from build123d import *

# Parameters (mm, degrees)
MODEL_R         = 1.59999954
EXTRUDE_1_DEPTH = 3.5
SKETCH_2_W      = 135.00000272
SKETCH_2_H      = 6
EXTRUDE_2_DEPTH = 3.5
FILLET_2_R      = 3
FILLET_3_R      = 3
FILLET_4_R      = 3
FILLET_5_R      = 3
FILLET_6_R      = 3
FILLET_7_R      = 3
FILLET_8_R      = 3
FILLET_9_R      = 3
FILLET_10_R     = 3
FILLET_11_R     = 3
FILLET_12_DEPTH = 3.5
FILLET_13_R     = 3
FILLET_14_R     = 3
FILLET_15_DEPTH = 3.5
FILLET_16_R     = 3
FILLET_17_R     = 3
SHELL_5_DEPTH   = 1.55


with BuildPart() as part:
    # Model → 凸台-拉伸1 (new body)
    with BuildSketch(Plane.XY):
        with BuildLine():
            Line((84.889976, 100), (147.00000318, 100))
            ThreePointArc((147.00000318, 100), (149.121322873, 99.121320613), (150.00000226, 97.00000092))
            Line((150.00000226, 97.00000092), (150.00000226, 3.00000162))
            ThreePointArc((150.00000226, 3.00000162), (149.121322873, 0.878681927), (147.00000318, 2.54e-06))
            Line((147.00000318, 2.54e-06), (2.99999908, 2.54e-06))
            ThreePointArc((2.99999908, 2.54e-06), (0.878679387, 0.878681927), (0, 3.00000162))
            Line((0, 3.00000162), (0, 97.00000092))
            ThreePointArc((0, 97.00000092), (0.878679387, 99.121320613), (2.99999908, 100))
            Line((2.99999908, 100), (66.109976, 100))
            ThreePointArc((66.109976, 100), (66.463529391, 99.853553391), (66.609976, 99.5))
            Line((66.609976, 99.5), (66.609976, 66))
            Line((66.609976, 66), (84.389976, 66))
            Line((84.389976, 66), (84.389976, 99.5))
            ThreePointArc((84.389976, 99.5), (84.536422609, 99.853553391), (84.889976, 100))
        make_face()
        with Locations((4.49999862, 95.50000204)):
            Circle(MODEL_R, mode=Mode.SUBTRACT)
        with Locations((145.5000138, 95.50001474)):
            Circle(MODEL_R, mode=Mode.SUBTRACT)
        with Locations((145.5000138, 4.49999608)):
            Circle(MODEL_R, mode=Mode.SUBTRACT)
        with Locations((4.49999354, 4.49999608)):
            Circle(MODEL_R, mode=Mode.SUBTRACT)
        with BuildLine():
            Line((59.609976, 58.5), (91.389976, 58.5))
            ThreePointArc((91.389976, 58.5), (91.743529391, 58.646446609), (91.889976, 59))
            Line((91.889976, 59), (91.889976, 92.00000066))
            ThreePointArc((91.889976, 92.00000066), (92.036422609, 92.353554051), (92.389976, 92.50000066))
            Line((92.389976, 92.50000066), (139.50000364, 92.50000066))
            ThreePointArc((139.50000364, 92.50000066), (141.621323333, 91.621321273), (142.50000272, 89.50000158))
            Line((142.50000272, 89.50000158), (142.50000272, 10.49999608))
            ThreePointArc((142.50000272, 10.49999608), (141.621323333, 8.378676387), (139.50000364, 7.499997))
            Line((139.50000364, 7.499997), (10.49999908, 7.499997))
            ThreePointArc((10.49999908, 7.499997), (8.378679387, 8.378676387), (7.5, 10.49999608))
            Line((7.5, 10.49999608), (7.5, 89.50000158))
            ThreePointArc((7.5, 89.50000158), (8.378679387, 91.621321273), (10.49999908, 92.50000066))
            Line((10.49999908, 92.50000066), (58.609976, 92.50000066))
            ThreePointArc((58.609976, 92.50000066), (58.963529391, 92.353554051), (59.109976, 92.00000066))
            Line((59.109976, 92.00000066), (59.109976, 59))
            ThreePointArc((59.109976, 59), (59.256422609, 58.646446609), (59.609976, 58.5))
        make_face(mode=Mode.SUBTRACT)
    extrude(amount=EXTRUDE_1_DEPTH)

    # 草图2 → 凸台-拉伸2 (add)
    with BuildSketch(Plane(origin=(0, 0, 0), x_dir=(-1, 0, 0), z_dir=(0, 0, -1))):
        with Locations((-75.00000136, 58.9994)):
            Rectangle(SKETCH_2_W, SKETCH_2_H)
        Polygon((-7.5, 30.00002482), (-65.0000272, 30.00002482), (-65.0000272, 7.499997), (-71.0000272, 7.499997), (-79.0000068, 7.499997), (-85.0000068, 7.499997), (-85.0000068, 30.00002482), (-142.50000272, 30.00002482), (-142.50000272, 36), (-7.5, 36), align=None)
    extrude(amount=-EXTRUDE_2_DEPTH)

    # 圆角2
    fillet_2_edges = [part.edges().sort_by_distance(p)[0] for p in [
        (142.50000272, 30.00002482, 1.75),
    ]]
    fillet(fillet_2_edges, radius=FILLET_2_R)

    # 圆角3
    fillet_3_edges = [part.edges().sort_by_distance(p)[0] for p in [
        (85.0000068, 30.00002482, 1.75),
    ]]
    fillet(fillet_3_edges, radius=FILLET_3_R)

    # 圆角4
    fillet_4_edges = [part.edges().sort_by_distance(p)[0] for p in [
        (85.0000068, 7.499997, 1.75),
    ]]
    fillet(fillet_4_edges, radius=FILLET_4_R)

    # 圆角5
    fillet_5_edges = [part.edges().sort_by_distance(p)[0] for p in [
        (65.0000272, 30.00002482, 1.75),
    ]]
    fillet(fillet_5_edges, radius=FILLET_5_R)

    # 圆角6
    fillet_6_edges = [part.edges().sort_by_distance(p)[0] for p in [
        (7.5, 30.00002482, 1.75),
    ]]
    fillet(fillet_6_edges, radius=FILLET_6_R)

    # 圆角7
    fillet_7_edges = [part.edges().sort_by_distance(p)[0] for p in [
        (65.0000272, 7.499997, 1.75),
    ]]
    fillet(fillet_7_edges, radius=FILLET_7_R)

    # 圆角8
    fillet_8_edges = [part.edges().sort_by_distance(p)[0] for p in [
        (7.5, 55.9994, 1.75),
    ]]
    fillet(fillet_8_edges, radius=FILLET_8_R)

    # 圆角9
    fillet_9_edges = [part.edges().sort_by_distance(p)[0] for p in [
        (7.5, 36, 1.75),
    ]]
    fillet(fillet_9_edges, radius=FILLET_9_R)

    # 圆角10
    fillet_10_edges = [part.edges().sort_by_distance(p)[0] for p in [
        (142.50000272, 55.9994, 1.75),
    ]]
    fillet(fillet_10_edges, radius=FILLET_10_R)

    # 圆角11
    fillet_11_edges = [part.edges().sort_by_distance(p)[0] for p in [
        (142.50000272, 36, 1.75),
    ]]
    fillet(fillet_11_edges, radius=FILLET_11_R)

    # 圆角12: read off the stored shape, not the designer's step
    # 圆角12 outline → 圆角12 (add)
    with BuildSketch(Plane.XY):
        with BuildLine():
            ThreePointArc((56.109976, 92.50000066), (58.231296344, 91.621321004), (59.109976, 89.50000066))
            Line((59.109976, 89.50000066), (59.109976, 92.00000066))
            ThreePointArc((59.109976, 92.00000066), (58.963529391, 92.353554051), (58.609976, 92.50000066))
            Line((58.609976, 92.50000066), (56.109976, 92.50000066))
        make_face()
    extrude(amount=FILLET_12_DEPTH)

    # 圆角13
    fillet_13_edges = [part.edges().sort_by_distance(p)[0] for p in [
        (7.5, 61.9994, 1.75),
    ]]
    fillet(fillet_13_edges, radius=FILLET_13_R)

    # 圆角14
    fillet_14_edges = [part.edges().sort_by_distance(p)[0] for p in [
        (59.109976, 61.9994, 1.75),
    ]]
    fillet(fillet_14_edges, radius=FILLET_14_R)

    # 圆角15: read off the stored shape, not the designer's step
    # 圆角15 outline → 圆角15 (add)
    with BuildSketch(Plane.XY):
        with BuildLine():
            ThreePointArc((91.889976, 89.50000066), (92.768655656, 91.621321004), (94.889976, 92.50000066))
            Line((94.889976, 92.50000066), (92.389976, 92.50000066))
            ThreePointArc((92.389976, 92.50000066), (92.036422609, 92.353554051), (91.889976, 92.00000066))
            Line((91.889976, 92.00000066), (91.889976, 89.50000066))
        make_face()
    extrude(amount=FILLET_15_DEPTH)

    # 圆角16
    fillet_16_edges = [part.edges().sort_by_distance(p)[0] for p in [
        (91.889976, 61.9994, 1.75),
    ]]
    fillet(fillet_16_edges, radius=FILLET_16_R)

    # 圆角17
    fillet_17_edges = [part.edges().sort_by_distance(p)[0] for p in [
        (142.50000272, 61.9994, 1.75),
    ]]
    fillet(fillet_17_edges, radius=FILLET_17_R)

    # 抽壳5: read off the stored shape, not the designer's step
    # 抽壳5 outline → 抽壳5 (cut)
    with BuildSketch(Plane.XY):
        with BuildLine():
            Line((148.05000226, 6.96982514), (148.05000226, 93.03018568))
            ThreePointArc((148.05000226, 93.03018568), (145.651621189, 91.953253974), (143.170088948, 92.821592272))
            ThreePointArc((143.170088948, 92.821592272), (144.118954267, 91.279829099), (144.45000272, 89.50000158))
            Line((144.45000272, 89.50000158), (144.45000272, 64.9994))
            ThreePointArc((144.45000272, 64.9994), (143.000181287, 61.499221433), (139.50000272, 60.0494))
            Line((139.50000272, 60.0494), (94.889976, 60.0494))
            ThreePointArc((94.889976, 60.0494), (91.389797433, 61.499221433), (89.939976, 64.9994))
            Line((89.939976, 64.9994), (89.939976, 89.50000066))
            ThreePointArc((89.939976, 89.50000066), (91.389797433, 93.000179227), (94.889976, 94.45000066))
            Line((94.889976, 94.45000066), (139.50000364, 94.45000066))
            ThreePointArc((139.50000364, 94.45000066), (141.279830004, 94.118952652), (142.821592497, 93.170088549))
            ThreePointArc((142.821592497, 93.170088549), (141.953252898, 95.651618945), (143.030181436, 98.05))
            Line((143.030181436, 98.05), (86.339976, 98.05))
            Line((86.339976, 98.05), (86.339976, 64.05))
            Line((86.339976, 64.05), (64.659976, 64.05))
            Line((64.659976, 64.05), (64.659976, 98.05))
            Line((64.659976, 98.05), (6.969817872, 98.05))
            ThreePointArc((6.969817872, 98.05), (8.046756275, 95.651682201), (7.178507736, 93.170176799))
            ThreePointArc((7.178507736, 93.170176799), (8.720234077, 94.118976296), (10.49999908, 94.45000066))
            Line((10.49999908, 94.45000066), (56.109976, 94.45000066))
            ThreePointArc((56.109976, 94.45000066), (59.610154567, 93.000179227), (61.059976, 89.50000066))
            Line((61.059976, 89.50000066), (61.059976, 64.9994))
            ThreePointArc((61.059976, 64.9994), (59.610154567, 61.499221433), (56.109976, 60.0494))
            Line((56.109976, 60.0494), (10.5, 60.0494))
            ThreePointArc((10.5, 60.0494), (6.999821433, 61.499221433), (5.55, 64.9994))
            Line((5.55, 64.9994), (5.55, 89.50000158))
            ThreePointArc((5.55, 89.50000158), (5.881024364, 91.279766583), (6.829823861, 92.821492924))
            ThreePointArc((6.829823861, 92.821492924), (4.348317985, 91.953244405), (1.95, 93.030183469))
            Line((1.95, 93.030183469), (1.95, 6.969819896))
            ThreePointArc((1.95, 6.969819896), (4.348331062, 8.046754491), (6.829840696, 7.178486133))
            ThreePointArc((6.829840696, 7.178486133), (5.881028875, 8.720219371), (5.55, 10.49999608))
            Line((5.55, 10.49999608), (5.55, 27.00002482))
            ThreePointArc((5.55, 27.00002482), (6.999821433, 30.500203387), (10.5, 31.95002482))
            Line((10.5, 31.95002482), (62.0000272, 31.95002482))
            ThreePointArc((62.0000272, 31.95002482), (65.500205767, 30.500203387), (66.9500272, 27.00002482))
            Line((66.9500272, 27.00002482), (66.9500272, 10.499997))
            ThreePointArc((66.9500272, 10.499997), (65.500205767, 6.999818433), (62.0000272, 5.549997))
            Line((62.0000272, 5.549997), (10.49999908, 5.549997))
            ThreePointArc((10.49999908, 5.549997), (8.720220238, 5.881026696), (7.178485744, 6.829840763))
            ThreePointArc((7.178485744, 6.829840763), (8.046751881, 4.348331965), (6.969817356, 1.95000254))
            Line((6.969817356, 1.95000254), (143.030189984, 1.95000254))
            ThreePointArc((143.030189984, 1.95000254), (141.953254903, 4.348344975), (142.821538688, 6.829860413))
            ThreePointArc((142.821538688, 6.829860413), (141.279796144, 5.881031961), (139.50000364, 5.549997))
            Line((139.50000364, 5.549997), (88.0000068, 5.549997))
            ThreePointArc((88.0000068, 5.549997), (84.499828233, 6.999818433), (83.0500068, 10.499997))
            Line((83.0500068, 10.499997), (83.0500068, 27.00002482))
            ThreePointArc((83.0500068, 27.00002482), (84.499828233, 30.500203387), (88.0000068, 31.95002482))
            Line((88.0000068, 31.95002482), (139.50000272, 31.95002482))
            ThreePointArc((139.50000272, 31.95002482), (143.000181287, 30.500203387), (144.45000272, 27.00002482))
            Line((144.45000272, 27.00002482), (144.45000272, 10.49999608))
            ThreePointArc((144.45000272, 10.49999608), (144.118969266, 8.720207487), (143.170144932, 7.178467247))
            ThreePointArc((143.170144932, 7.178467247), (145.651658255, 8.046755262), (148.05000226, 6.96982514))
        make_face()
        with BuildLine():
            Line((144.45000272, 52.9994), (144.45000272, 39))
            ThreePointArc((144.45000272, 39), (143.000181287, 35.499821433), (139.50000272, 34.05))
            Line((139.50000272, 34.05), (10.5, 34.05))
            ThreePointArc((10.5, 34.05), (6.999821433, 35.499821433), (5.55, 39))
            Line((5.55, 39), (5.55, 52.9994))
            ThreePointArc((5.55, 52.9994), (6.999821433, 56.499578567), (10.5, 57.9494))
            Line((10.5, 57.9494), (139.50000272, 57.9494))
            ThreePointArc((139.50000272, 57.9494), (143.000181287, 56.499578567), (144.45000272, 52.9994))
        make_face(mode=Mode.SUBTRACT)
    extrude(amount=SHELL_5_DEPTH, mode=Mode.SUBTRACT)


solid = part.part
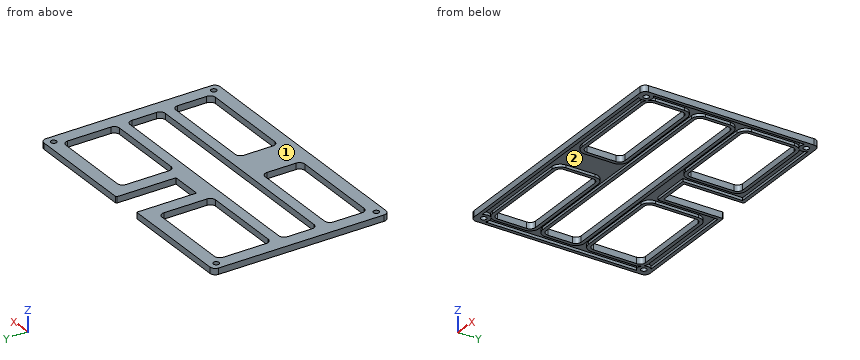
Verification items for the finished model (mm, model axes). Face numbers are marked on the shaded views. Coordinates: 2 decimals unless noted, no trailing zeros. Loops run counter-clockwise (first coordinate to the right, second up) from the corner with the lowest first, then second, coordinate; pieces in that order, holes last. Notation, with made-up numbers: M 87.25,71.25 L 101.25,71.25 A36 cw 101.25,109.25 Z; hole C 44,-33 d2. An arc over 180 degrees is marked long. One line per item, written item: value.
1. Material ranges on line 1 along Y through (x, z) = (117, 2.8); line 2 along X through (y, z) = (83.5, 3.1); line 3 along X through (y, z) = (16, 0.8), recorded low to high. Write a range as from..to.
Answers follow:
line 1: 0..7.5, 30..36, 56..62, 92.5..100
line 2: 0..7.5, 59.11..66.61, 84.39..91.89, 142.5..150
line 3: 0..1.95, 5.55..7.5, 65..66.95, 83.05..85, 142.5..144.45, 148.05..150
2. Section check D-D on x = 75. Record the cut outline in (y, z).
Answers follow:
outline: M 0,0 L 1.95,0 L 1.95,1.55 L 34.05,1.55 L 34.05,0 L 36,0 L 36,3.5 L 0,3.5 Z; M 56,0 L 57.95,0 L 57.95,1.55 L 64.05,1.55 L 64.05,0 L 66,0 L 66,3.5 L 56,3.5 Z
3. Section check A-A on y = 77.5. Give the number of separate pieces and of enclosed holes in the cut face, plus the area to 3 significant figures.
Answers follow:
separate pieces: 4
enclosed holes: 0
area: 82.7 mm^2
4. Mould release check, pull along X, two halves, no side actions. Record for the marked faces 1 and 2: pulls with the +X half, pulls with the -X half, needs draft (parallel to the pull), parting line crosses it, or undercut.
Answers follow:
face 1: needs draft
face 2: undercut
5. Gauge pin test, flat end, axial feed: P1, Ø0.8, axis at x = 68, z = 1, coming from the +Y side. Record the tip position at first contact, or that the pin passes through.
Answers follow:
P1: y = 66
6. Section check C-C on y = 16. Record the cut outline in (x, z).
Answers follow:
outline: M 0,0 L 1.95,0 L 1.95,1.55 L 5.55,1.55 L 5.55,0 L 7.5,0 L 7.5,3.5 L 0,3.5 Z; M 65,0 L 66.95,0 L 66.95,1.55 L 83.05,1.55 L 83.05,0 L 85,0 L 85,3.5 L 65,3.5 Z; M 142.5,0 L 144.45,0 L 144.45,1.55 L 148.05,1.55 L 148.05,0 L 150,0 L 150,3.5 L 142.5,3.5 Z
